from build123d import *

# Parameters (mm, degrees)
F0_W        = 15.3297632933
F0_H        = 43.554501608
F0_W_2      = 41.3750298321
F0_W_3      = 28.9361141622
F1_DEPTH    = 25.4
F2_W        = 17.5558461342
F2_H        = 43.554501608
F3_DEPTH    = 25.4
F4_SIZE     = 15.24
F5_T4_DEPTH = 174.1959973967
F6_DEPTH    = 12.7
F7_DEPTH    = 25.4
F8_DEPTH    = 12.7


# Not quite as in the source:
# - a fillet or chamfer that OpenCascade refuses, or shapes differently, is made with other operations: its cross-section is extruded or revolved along the edge and cut away or added


with BuildPart() as f1:
    # F0 (on Top) → F1 (new body)
    with BuildSketch(Plane.XY):
        with Locations((-7.6648816466, -1.5181871131)):
            Rectangle(F0_W, F0_H)
        with Locations((20.6875149161, -1.5181871131)):
            Rectangle(F0_W_2, F0_H)
        with Locations((55.8430869132, -1.5181871131)):
            Rectangle(F0_W_3, F0_H)
    extrude(amount=F1_DEPTH)

    # F2 (on face) → F3 (join)
    with BuildSketch(Plane.XY.offset(25.4)):
        with Locations((-6.5518402262, -1.5181871131)):
            Rectangle(F2_W, F2_H)
    extrude(amount=F3_DEPTH)

    # F4
    f4_edges = [f1.edges().sort_by_distance(p)[0] for p in [
        (70.311144, -1.518187, 25.4),
    ]]
    chamfer(f4_edges, length=F4_SIZE)

    # F5: chamfer of 25.4 on 1 edges, made by hand


with BuildPart() as f5_tool2:
    # F5_s3 → F5_t4 (new body)
    with BuildSketch(Plane.XZ.offset(88.6161858114)):
        Polygon((2.2260828409, 25.4), (-23.1739171591, 50.8), (2.2260828409, 50.8), align=None)
    extrude(amount=-F5_T4_DEPTH)

    split(bisect_by=Plane.XY.offset(25.4), keep=Keep.TOP)


with BuildPart() as f1_1:
    add(f1.part)

    # F5_t1: cut F5_tool2
    add(f5_tool2.part, mode=Mode.SUBTRACT)

    # F6 (add): a face of the model
    f6_faces = [f1_1.faces().sort_by_distance(p)[0] for p in [
        (-15.3297632933, -1.5181871131, 21.4779230671),
    ]]
    extrude(f6_faces, amount=F6_DEPTH)

    # F7 (add): a face of the model
    f7_faces = [f1_1.faces().sort_by_distance(p)[0] for p in [
        (14.1137713258, 20.2590636909, 15.1513351417),
    ]]
    extrude(f7_faces, amount=F7_DEPTH)

    # F8 (add): a face of the model
    f8_faces = [f1_1.faces().sort_by_distance(p)[0] for p in [
        (14.1137713258, 45.6590636909, 15.1513351417),
    ]]
    extrude(f8_faces, amount=F8_DEPTH)


solid = f1_1.part
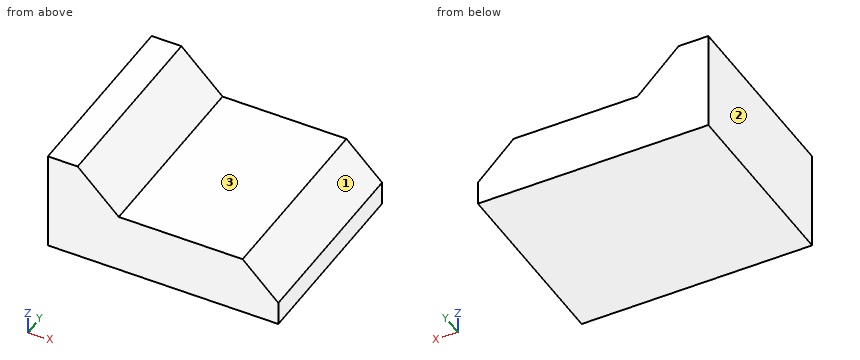
Could you check a few things on this model? Use its own coordinates, in mm. Face numbers are marked on the shaded views. Coordinates: 2 decimals unless noted, no trailing zeros. Order: outer loops, then holes, each group sorted by start corner. A loop starts at its lowest first (then second) coordinate and runs counter-clockwise, first axis right, second up.
Q1. Suppose I cut it at A-A on y = 7. Please give me the cut outline in (x, z), and give its area (3 significant figures).
Q2. Will these pins go through, and if not, where does the flat tip stop? pin 1 (4 mm diameter, centred on x = 27.5, y = 7, fed in from -Z); pin 2 (1 mm diameter, centred on x = 39.5, y = 9, fed in from +Z).
Q3. Thinking about a two-plate mould opening in X: for the marked faces 1, 2 and 3, which applies, released by +X, released by -X, zero draft, split by the parting line, or undercut?
Q4. Suppose I cut it at B-B on x = 25. Please give me the cut outline in (y, z).
Q5. Please list where these lines run through material, in increasing order: L1, parallel to Z at x = 19, y = 37; L2, parallel to Z at x = -14, y = 4; L3, parallel to X at y = -16.5, z = 21.5.
Q6. Suppose I cut it at C-C on z = 33. Please give me the cut outline in (x, y).
Answer:
1. outline: (-28.03, 0) - (70.31, 0) - (70.31, 10.16) - (55.07, 25.4) - (2.23, 25.4) - (-15.33, 42.96) - (-28.03, 42.96) - close
1. area: 2,760 mm2
2. pin 1: stops at z = 0
2. pin 2: stops at z = 25.4
3. face 1: released by +X
3. face 2: released by -X
3. face 3: zero draft
4. outline: (-23.3, 0) - (58.36, 0) - (58.36, 25.4) - (-23.3, 25.4) - close
5. L1: z = 0 to 25.4
5. L2: z = 0 to 41.63
5. L3: x = -28.03 to 58.97
6. outline: (-28.03, -23.3) - (-5.37, -23.3) - (-5.37, 58.36) - (-28.03, 58.36) - close
